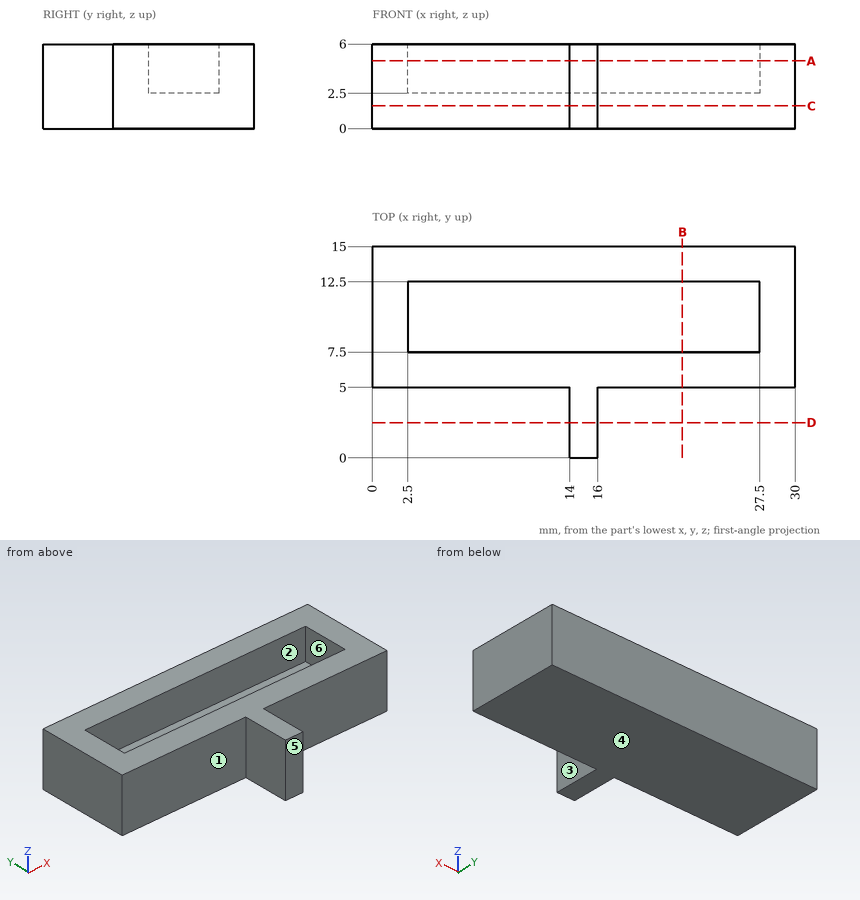
Check sheet for the drawn part. Datum: minimum x, y, z corner. Units: mm. A direction names the side the tool comes from. Round coordinates to 2 decimals unless told otherwise and drop trailing zeros. Write each loop counter-clockwise with the first axis right and the second up, starting at its lowest first coordinate (ties: lowest second). Pieces come first, ordered by that corner, then holes. Notation, with made-up numbers: (40, 63.25) -> (63, 63.25) arc R19 cw to (63, 95.25) -> close; hole circle Ø9 at (84.5, 56.5). An arc over 180 degrees is marked (long way). One line per item, written item: value. Start each with the question number.
(1) Cross-section at B-B, the plane x = 22. Record the cut outline in (y, z), and give its area (3 significant figures).
(2) Draft check along Y on the marked faces 4, 5 and 6. Enter one of: +Y half, -Y half, draft (parallel to the pull), parting line (faces both ways), or undercut.
(3) Go/stop test with flat-tipped pins: pin 1 Ø3 at (x, z) = (10.5, 5) entering from -Y; pin 2 Ø1.5 at (y, z) = (2.5, 2.5) entering from +X; pin 3 Ø2.5 at (x, y) = (10, 9) entering from +Z. Record where each tip stops, or that it passes through.
(4) Cross-section at C-C, the plane z = 1.6. Record the cut outline in (x, y), and give its area (3 significant figures).
(5) Access from +Z, -Z, +X, -X, +Y, -Y to the whole of each face (thin tool, end or side, straight path). Record for the marked faces 1, 2 and 3.
(6) Scan lines: line 1 (Y direction, x = 25.5, z = 5.4); line 2 (X direction, y = 7.75, z = 5.6); line 3 (X direction, y = 3.75, z = 4.7). Record each from-to range of solid material in increasing order. Write a range as [from, to].
(7) Cross-section at D-D, the plane y = 2.5. Record the cut outline in (x, z), and give its area (3 significant figures).
(8) Cross-section at A-A, the plane z = 4.8. Record the cut outline in (x, y), and give its area (3 significant figures).
Answer:
1. outline: (5, 0) -> (15, 0) -> (15, 6) -> (12.5, 6) -> (12.5, 2.5) -> (7.5, 2.5) -> (7.5, 6) -> (5, 6) -> close
1. area: 42.5 mm²
2. face 4: draft
2. face 5: -Y half
2. face 6: undercut
3. pin 1: y = 5
3. pin 2: x = 16
3. pin 3: z = 2.5
4. outline: (0, 5) -> (14, 5) -> (14, 0) -> (16, 0) -> (16, 5) -> (30, 5) -> (30, 15) -> (0, 15) -> close
4. area: 310 mm²
5. face 1: +Z, -Z, -X, -Y
5. face 2: +Z
5. face 3: +Z, -Z, +X, -Y
6. line 1: [5, 7.5], [12.5, 15]
6. line 2: [0, 2.5], [27.5, 30]
6. line 3: [14, 16]
7. outline: (14, 0) -> (16, 0) -> (16, 6) -> (14, 6) -> close
7. area: 12.0 mm²
8. outline: (0, 5) -> (14, 5) -> (14, 0) -> (16, 0) -> (16, 5) -> (30, 5) -> (30, 15) -> (0, 15) -> close; hole (2.5, 7.5) -> (27.5, 7.5) -> (27.5, 12.5) -> (2.5, 12.5) -> close
8. area: 185 mm²
